Check sheet for the modelled part. Datum: model origin and axes. Units: mm. A direction names the side the tool comes from. Round coordinates to 2 decimals unless told otherwise and drop trailing zeros. Loops run counter-clockwise (first coordinate to the right, second up) from the corner with the lowest first, then second, coordinate; pieces in that order, holes last. Notation, with made-up numbers: (-24.75, 4) - (4.25, 4) arc R30 cw to (4.25, 32) - close; hole circle Ø8 at (29, -13). An arc over 180 degrees is marked (long way). Put each result on its own line as item: value.
```python
from build123d import *

# Parameters (mm, degrees)
SKETCH1_R           = 16
BOSS_EXTRUDE1_DEPTH = 20
SKETCH3_W           = 25
SKETCH3_H           = 1
CIRPATTERN1_COUNT   = 3


with BuildPart() as part:
    # Sketch1 → Boss-Extrude1 (new body)
    with BuildSketch(Plane(origin=(0, 0, 0), x_dir=(1, 0, 0), z_dir=(0, 1, 0))):
        with Locations(Location((0, 0, 0), (0, 0, 270))):
            Circle(SKETCH1_R)
        with BuildLine():
            Line((-1, -12), (1, -12))
            Line((1, -12), (1, -13.964240044))
            ThreePointArc((1, -13.964240044), (0, 14), (-1, -13.964240044))
            Line((-1, -13.964240044), (-1, -12))
        make_face(mode=Mode.SUBTRACT)
    extrude(amount=BOSS_EXTRUDE1_DEPTH)

    # Sweep1: sweep along a curve in space
    with BuildLine() as sweep1_path:
        add(Edge.make_bspline(
            [(0, 0, 16), (-1.857798397, 2.217583486, 16), (-5.586575728, 6.669449908, 15.343093774), (-10.494221117, 13.330550092, 12.509663387), (-12.927507262, 17.782416514, 9.608900607), (-13.856406461, 20, 8)],
            knots=[0, 0, 0, 0, 0.333333333, 0.666666667, 1, 1, 1, 1], degree=3))
    with BuildLine() as sweep1_axis:
        Line((0, 0, 0), (0, 20, 0))
    # Sketch3 → Sweep1 (sweep)
    with BuildSketch(Plane(origin=(0, 0, 0), x_dir=(0, 0, -1), z_dir=(1, 0, 0))):
        with Locations((-28.5, 0.5)):
            Rectangle(SKETCH3_W, SKETCH3_H)
    sweep1 = sweep(path=sweep1_path.line, binormal=sweep1_axis.edges()[0])

    # CirPattern1: Sweep1 ×3 about axis
    cirpattern1_axis = Axis((0, -1.105625, 0), (0, 1, 0))
    for i in range(1, CIRPATTERN1_COUNT):
        add(sweep1.rotate(cirpattern1_axis, i * 360 / CIRPATTERN1_COUNT))


solid = part.part
```
Item 1: Release check for a two-part mould opening along X. For faces 1 (the flat face through (0, 0, 13)), 2 (the cylindrical face through (-16, 10, 0)), 3 (the flat face through (1, 10, 13)), 4 (the cylindrical face through (0.602, 9.86, -13.987)) record: +X half, -X half, draft (parallel to the pull), parting line (faces both ways), or undercut.
Filled sheet:
face 1: draft
face 2: -X half
face 3: undercut
face 4: undercut
Item 2: Tool access check on faces 5 (the flat face through (0, 10, 12)), 6 (the flat face through (-24.833, 20.507, 14.337)), 7 (the flat face through (24.53, 0.493, -14.162)), 8 (the flat face through (24.833, 20.507, 14.338)). Record the directions out of +Z, -Z, +X, -X, +Y, -Y that give a thin tool (end or side, any length) a straight path to the whole face; none if there is none.
Filled sheet:
face 5: +Y, -Y
face 6: -Z, -X, +Y, -Y
face 7: -Z, +Y, -Y
face 8: +Z, +Y, -Y
Item 3: Section check A-A on x = 2. Enter the section's corners in (y, z).
Filled sheet:
outline: (0, -15.87) - (20, -15.87) - (20, -13.86) - (0, -13.86) - close; (0, 13.86) - (20, 13.86) - (20, 15.87) - (0, 15.87) - close
Item 4: Go/stop test with flat-tipped pins: pin 1 (1.5 mm diameter, centred on x = 31, z = 10, fed in from -Y); pin 2 (3 mm diameter, centred on x = 28, y = 9, fed in from -Z); pin 3 (10 mm diameter, centred on x = -22.5, y = 9.5, fed in from -Z). Record where each tip stops, or that it passes through.
Filled sheet:
pin 1: y = 15.52
pin 2: z = -5.21
pin 3: z = -36.9
Item 5: Section check B-B on z = 10.5. Count the separate pieces of the cut face and the enclosed holes in it, then the cut area to 3 significant figures.
Filled sheet:
separate pieces: 3
enclosed holes: 0
area: 140 mm²
Item 6: Thickness scan on line 1 (X direction, y = 12.5, z = 0); line 2 (Y direction, x = -8.5, z = -12); line 3 (Z direction, x = 4.5, y = 10.75). Record the ranges inside material, lowest first. Write a range as from..to.
Filled sheet:
line 1: -16..-14, 14..16
line 2: 0..20
line 3: -15.35..-13.26, 13.26..15.35
